from build123d import *

# Parameters (mm, degrees)
F0_W     = 30
F0_H     = 5
F1_DEPTH = 5


with BuildPart() as f1:
    # F0 (on Right) → F1 (new body)
    with BuildSketch(Plane.YZ):
        with BuildLine():
            ThreePointArc((-5, 0), (-1.464466, 1.464466), (0, 5))
            Line((0, 5), (0, 50))
            Line((0, 50), (42, 50))
            Line((42, 50), (42, 5))
            ThreePointArc((42, 5), (43.464466, 1.464466), (47, 0))
            Line((47, 0), (97, 0))
            ThreePointArc((97, 0), (100.535534, 1.464466), (102, 5))
            Line((102, 5), (102, 10.837785))
            ThreePointArc((102, 10.837785), (101.589267, 12.822382), (100.42455, 14.480923))
            Line((100.42455, 14.480923), (53.44347, 58.643138))
            ThreePointArc((53.44347, 58.643138), (51.8607, 59.648424), (50.01892, 60))
            Line((50.01892, 60), (-8.01892, 60))
            ThreePointArc((-8.01892, 60), (-9.8607, 59.648424), (-11.44347, 58.643138))
            Line((-11.44347, 58.643138), (-58.42455, 14.480923))
            ThreePointArc((-58.42455, 14.480923), (-59.589267, 12.822382), (-60, 10.837785))
            Line((-60, 10.837785), (-60, 5))
            ThreePointArc((-60, 5), (-58.535534, 1.464466), (-55, 0))
            Line((-55, 0), (-5, 0))
        make_face()
        with Locations((-30, 10.5)):
            Rectangle(F0_W, F0_H, mode=Mode.SUBTRACT)
        with Locations((72, 10.5)):
            Rectangle(F0_W, F0_H, mode=Mode.SUBTRACT)
    extrude(amount=F1_DEPTH)


solid = f1.part
The listing builds one solid part. Answer for the finished solid, in the listing's coordinates (mm). A direction names the side the tool comes from. Coordinates: 2 decimals unless noted, no trailing zeros. Order: outer loops, then holes, each group sorted by start corner. A loop starts at its lowest first (then second) coordinate and runs counter-clockwise, first axis right, second up.
Q1. A cutting plane is placed at C-C, the plane x = 2.7. Write down the section's boundary in (y, z), and give its area (3 significant figures).
Q2. Consider line 1 (Y direction, x = 4.6, z = 10); line 2 (Y direction, x = 2.75, z = 4.5); line 3 (Z direction, x = 4.45, y = 6). Determine where each line is inside the solid, lowest interval first.
Q3. Given P1, Ø2.5, axis at x = 1.5, z = 35, coming from the +Y side; P2, Ø2, axis at x = 2.5, y = 28, coming from the -Z side; P3, Ø3, axis at x = 4, z = 29, coming from the +Y side, each flat-ended and moving along its own axis, determine where each tip first touches the part or whether it passes through.
Q4. Which of the six approach directions +Z, -Z, +X, -X, +Y, -Y give full straight-line access (tool end or side, diameter ignored) to faces 4 (the face through (2, 100, 1)), 5 (the face through (2, 42, 28)), 6 (the face through (2, 57, 10))?
Q5. A cutting plane is placed at B-B, the plane z = 47.5. Write down the section's boundary in (x, y).
Q6. A cutting plane is placed at A-A, the plane y = 61. Write down the section's boundary in (x, z), and give its area (3 significant figures).
Q7. For a pull along Z with two mould halves and no side action, classify faces 1 (the face through (2, 21, 50)), 2 (the face through (5, 19.9, 50.4)), 3 (the face through (2, 72, 8)) as pulls with the +Z half, pulls with the -Z half, needs draft (parallel to the pull), parting line crosses it, or undercut.
Answers follow:
1. outline: (-60, 5) arc R5 ccw to (-55, 0) - (-5, 0) arc R5 ccw to (0, 5) - (0, 50) - (42, 50) - (42, 5) arc R5 ccw to (47, 0) - (97, 0) arc R5 ccw to (102, 5) - (102, 10.84) arc R5 ccw to (100.42, 14.48) - (53.44, 58.64) arc R5 ccw to (50.02, 60) - (-8.02, 60) arc R5 ccw to (-11.44, 58.64) - (-58.42, 14.48) arc R5 ccw to (-60, 10.84) - close; hole (-45, 8) - (-15, 8) - (-15, 13) - (-45, 13) - close; hole (57, 8) - (87, 8) - (87, 13) - (57, 13) - close
1. area: 4,950 mm2
2. line 1: y = -60 to -45, -15 to 0, 42 to 57, 87 to 102
2. line 2: y = -59.97 to -0.03, 42.03 to 101.97
2. line 3: z = 50 to 60
3. P1: stops at y = 79.93
3. P2: stops at z = 50
3. P3: stops at y = 86.57
4. face 4: -Z, +X, -X, +Y
4. face 5: -Z, +X, -X
4. face 6: +X, -X
5. outline: (0, -23.3) - (5, -23.3) - (5, 0) - (0, 0) - close; (0, 42) - (5, 42) - (5, 65.3) - (0, 65.3) - close
6. outline: (0, 0) - (5, 0) - (5, 8) - (0, 8) - close; (0, 13) - (5, 13) - (5, 51.54) - (0, 51.54) - close
6. area: 233 mm2
7. face 1: pulls with the -Z half
7. face 2: needs draft
7. face 3: undercut
